Can you work these out from the drawing? Everything is in mm from the part's minimum corner. A direction names the side the tool comes from. Round coordinates to 2 decimals unless told otherwise and drop trailing zeros. Loops run counter-clockwise (first coordinate to the right, second up) from the corner with the lowest first, then second, coordinate; pieces in that order, holes last. Notation, with made-up numbers: (-0.75, 57) -> (40.25, 57) arc R14 ccw to (40.25, 70) -> close; hole circle Ø2 at (52, 64). An arc over 180 degrees is marked (long way). Answer as a JSON object with one key per item and string values.
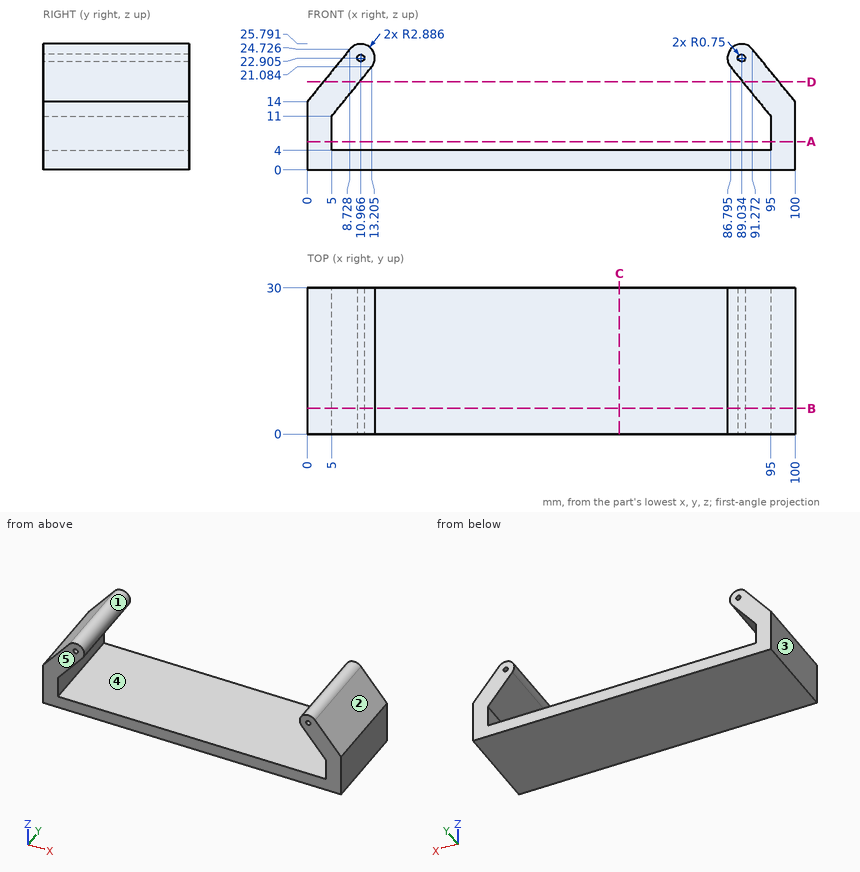
Q1. On a 3-axis mill with a long thin cutter (end or side, diameter ignored), from which of +Z, -Z, +X, -X, +Y, -Y can I reach the whole of each face in a straight line? I mean the marked faces 4 and 5. Say none if no direction works.
Determined:
{"face 4": "+Y, -Y", "face 5": "+Z, -Z, +X, -X, -Y"}
Q2. I want a section at C-C, the plane x = 64. Write out the boundary of the cut face in (y, z).
Determined:
{"outline": "(0, 0) -> (30, 0) -> (30, 4) -> (0, 4) -> close"}
Q3. I want a section at D-D, the plane z = 18. Write out the boundary of the cut face in (x, y) (1 decimal).
Determined:
{"outline": "(3.3, 0) -> (10.7, 0) -> (10.7, 30) -> (3.3, 30) -> close; (89.3, 0) -> (96.7, 0) -> (96.7, 30) -> (89.3, 30) -> close"}
Q4. I'm going to push flat-ended pins straight in: pin 1 (1 mm diameter, centred on x = 15.5, y = 14.5, fed in from +Z); pin 2 (12 mm diameter, centred on y = 25.5, z = 21, fed in from -X) (1 decimal); pin 3 (12 mm diameter, centred on x = 68, y = 8.5, fed in from -Z); pin 4 (5 mm diameter, centred on y = 20.5, z = 19.5, fed in from -X). Where does each tip first touch, or does it pass through?
Determined:
{"pin 1": "z = 4", "pin 2": "x = 0.8", "pin 3": "z = 0", "pin 4": "x = 2.44"}
Q5. I want a section at B-B, the plane y = 5.25. Give the number of separate pieces and of enclosed holes in the cut face.
Determined:
{"separate pieces": "1", "enclosed holes": "2"}
Q6. We'd pull the mould along Z, two halves only. Please class the marked faces 1, 2 and 3: pulls with the +Z half, pulls with the -Z half, needs draft (parallel to the pull), parting line crosses it, or undercut.
Determined:
{"face 1": "undercut", "face 2": "pulls with the +Z half", "face 3": "needs draft"}
Q7. I want a section at A-A, the plane z = 5.75. Write out the boundary of the cut face in (x, y).
Determined:
{"outline": "(0, 0) -> (5, 0) -> (5, 30) -> (0, 30) -> close; (95, 0) -> (100, 0) -> (100, 30) -> (95, 30) -> close"}
Q8. If I drill on L1, parallel to X at y = 4.75, z = 10.75; L2, parallel to X at y = 18, z = 23.5 (1 decimal); L3, parallel to Z at x = 56, y = 7.5, over which ranges is the centre line in solid material (lowest first)? Write a range as [from, to].
Determined:
{"L1": "[0, 5], [95, 100]", "L2": "[7.7, 10.5], [11.4, 13.8], [86.2, 88.6], [89.5, 92.3]", "L3": "[0, 4]"}
